Verification items for the finished model (mm, model axes). A direction names the side the tool comes from. Give positions to 0.01 mm unless a question says otherwise; leave off trailing zeros. Loops run counter-clockwise (first coordinate to the right, second up) from the corner with the lowest first, then second, coordinate; pieces in that order, holes last. Notation, with made-up numbers: M -13,15 L 8,15 A29 ccw 8,42 Z; hole C 11.25,-17.5 d2. An arc over 180 degrees is marked long. Use a Markdown table: item, result.
from build123d import *

# Parameters (mm, degrees)
F1_DEPTH = 12.7
F3_START = -6.35
F2_W     = 10.1600005239
F2_H     = 12.7
F3_DEPTH = 12.7
F5_START = -6.35
F4_W     = 6.35
F4_H     = 6.35
F5_DEPTH = 12.7


with BuildPart() as f1:
    # F0 (on Front) → F1 (new body, symmetric)
    with BuildSketch(Plane.XZ):
        Polygon((0, 25.4), (0, 0), (38.1, 0), (38.1, 12.7), (6.35, 12.7), (6.35, 25.4), align=None)
    extrude(amount=F1_DEPTH, both=True)

    # F2 (on face) → F3 (cut)
    with BuildSketch(Plane.XZ.offset(12.7).offset(F3_START)):
        with Locations((33.019999738, 6.35)):
            Rectangle(F2_W, F2_H)
    extrude(amount=-F3_DEPTH, mode=Mode.SUBTRACT)

    # F4 (on face) → F5 (cut)
    with BuildSketch(Plane.XZ.offset(12.7).offset(F5_START)):
        with Locations((3.175, 22.225)):
            Rectangle(F4_W, F4_H)
    extrude(amount=-F5_DEPTH, mode=Mode.SUBTRACT)


solid = f1.part
(1) Set-up check for faces 4 (the flat face through (27.94, 0, 6)), 5 (the flat face through (19, 0, 0)), 6 (the flat face through (15, 12.7, 7)), 7 (the flat face through (6.35, 0, 18)), 8 (the flat face through (3, -6.35, 22)): record each of +Z, -Z, +X, -X, +Y, -Y from which the full face is reachable in a straight line by a thin tool's end or side.
Results below:
| item | result |
|---|---|
| face 4 | +Z, -Z, +X |
| face 5 | -Z, +X, -X, +Y, -Y |
| face 6 | +Z, -Z, +X, -X, +Y |
| face 7 | +Z, +X, +Y, -Y |
| face 8 | +Z, +X, -X |
(2) Cross-section at D-D on y = -5.75. Record the cut outline in (x, z).
Results below:
| item | result |
|---|---|
| outline | M 0,0 L 27.94,0 L 27.94,12.7 L 6.35,12.7 L 6.35,19.05 L 0,19.05 Z |
(3) Cross-section at B-B on x = 4.5. Record the cut outline in (y, z), then the cut area to 3 significant figures.
Results below:
| item | result |
|---|---|
| outline | M -12.7,0 L 12.7,0 L 12.7,25.4 L 6.35,25.4 L 6.35,19.05 L -6.35,19.05 L -6.35,25.4 L -12.7,25.4 Z |
| area | 565 mm^2 |
(4) Cross-section at A-A on z = 21.5. Record the cut outline in (x, y).
Results below:
| item | result |
|---|---|
| outline | M 0,-12.7 L 6.35,-12.7 L 6.35,-6.35 L 0,-6.35 Z; M 0,6.35 L 6.35,6.35 L 6.35,12.7 L 0,12.7 Z |
(5) Cross-section at C-C on z = 6. Record the cut outline in (x, y).
Results below:
| item | result |
|---|---|
| outline | M 0,-12.7 L 38.1,-12.7 L 38.1,-6.35 L 27.94,-6.35 L 27.94,6.35 L 38.1,6.35 L 38.1,12.7 L 0,12.7 Z |
(6) Draft check along Y on faces 1 (the flat face through (33, 6.35, 6)), 2 (the flat face through (15, -12.7, 7)), 3 (the flat face through (38.1, 9, 6)). Enter one of: +Y half, -Y half, draft (parallel to the pull), parting line (faces both ways), or undercut.
Results below:
| item | result |
|---|---|
| face 1 | undercut |
| face 2 | -Y half |
| face 3 | draft |
(7) Material ranges on line 1 (Y direction, x = 35, z = 9.5); line 2 (Z direction, x = 11.5, y = 6); line 3 (X direction, y = 11.25, z = 15.25), recorded low to high.
Results below:
| item | result |
|---|---|
| line 1 | -12.7 to -6.35, 6.35 to 12.7 |
| line 2 | 0 to 12.7 |
| line 3 | 0 to 6.35 |
(8) Gauge pin test, flat ends, axial feed: P1, Ø6.5, axis at y = 0.5, z = 21, coming from the +X side; P2, Ø7.5, axis at x = 22.5, y = -6, coming from the +Z side; P3, Ø7, axis at x = 2, y = -0.5, coming from the +Z side. Record the tip position at first contact, or that the pin passes through.
Results below:
| item | result |
|---|---|
| P1 | x = 6.35 |
| P2 | z = 12.7 |
| P3 | z = 19.05 |
